For this review, take the finished solid that the model builds, in its own axes (mm). Coordinates: 2 decimals unless noted, no trailing zeros. Put each result on its own line as item: value. Start each with the question number.
Item 1: The part is to be moulded in two halves that separate along Z. For faces 1 (the flat face through (126, 4, -137)), 2 (the conical face through (49.11, 1.7, -162.32)), say which applies: +Z half, -Z half, draft (parallel to the pull), parting line (faces both ways), or undercut.
Item 2: To check wall thickness, follow L1, parallel to X at y = 0.85, z = -165; L2, parallel to X at y = 1.75, z = -135; L3, parallel to Z at x = 113, y = 0.6. State the ranges of each line that lie inside material, in increasing order.
Item 3: Insertion check: P1, Ø5, axis at x = 208, z = -165, coming from the +Y side. The pin has a flat end and moves straight along its axis. Give the tip position at first contact, or say it passes through.
```python
from build123d import *

# Parameters (mm, degrees)
SKETCH1_W                                      = 256
SKETCH1_H                                      = 270
BOSS_EXTRUDE1_DEPTH                            = 4
CSK_FOR_M5_FLAT_HEAD_MACHINE_SCREW1_AT_2_COUNT = 2
CSK_FOR_M5_FLAT_HEAD_MACHINE_SCREW1_AT_2_PITCH = 124.197423484
CSK_FOR_M5_FLAT_HEAD_MACHINE_SCREW1_AT_3_COUNT = 2
CSK_FOR_M5_FLAT_HEAD_MACHINE_SCREW1_AT_3_PITCH = 103.07764064
M6_TAPED_HOLE_THRMOCOUPLER_D                   = 5


with BuildPart() as part:
    # Sketch1 → Boss-Extrude1 (new body)
    with BuildSketch(Plane(origin=(0, 0, 0), x_dir=(1, 0, 0), z_dir=(0, 1, 0))):
        with Locations((128, 135)):
            Rectangle(SKETCH1_W, SKETCH1_H)
    extrude(amount=BOSS_EXTRUDE1_DEPTH)

    # Sketch2 → CSK for M5 Flat Head Machine Screw1 (revolve, cut)
    with BuildSketch(Plane(origin=(113, 4, -85), x_dir=(0, 0, 1), z_dir=(1, 0, 0))):
        Polygon((0, 0), (0, 4), (2.75, 4), (2.75, 2.45), (5.2, 0), align=None)
    csk_for_m5_flat_head_machine_screw1 = revolve(axis=Axis((113, 10.35, -85), (0, -1, 0)), mode=Mode.SUBTRACT)

    # CSK for M5 Flat Head Machine Screw1 at 2: CSK for M5 Flat Head Machine Screw1 ×2
    with Locations(*[Vector(0.7649111981170511, 0, -0.6441357457827795) * (i * CSK_FOR_M5_FLAT_HEAD_MACHINE_SCREW1_AT_2_PITCH) for i in range(1, CSK_FOR_M5_FLAT_HEAD_MACHINE_SCREW1_AT_2_COUNT)]):
        add(csk_for_m5_flat_head_machine_screw1, mode=Mode.SUBTRACT)

    # CSK for M5 Flat Head Machine Screw1 at 3: CSK for M5 Flat Head Machine Screw1 ×2
    with Locations(*[Vector(-0.6305926250944657, 0, -0.7761140001162656) * (i * CSK_FOR_M5_FLAT_HEAD_MACHINE_SCREW1_AT_3_PITCH) for i in range(1, CSK_FOR_M5_FLAT_HEAD_MACHINE_SCREW1_AT_3_COUNT)]):
        add(csk_for_m5_flat_head_machine_screw1, mode=Mode.SUBTRACT)

    # M6 taped hole - thrmocoupler (through all)
    with Locations(Plane(origin=(0, 4, 0), x_dir=(-1, 0, 0), z_dir=(0, 1, 0))):
        with Locations((-128, -135)):
            Hole(M6_TAPED_HOLE_THRMOCOUPLER_D / 2)


solid = part.part
```
Return value:
1. face 1: draft
1. face 2: undercut
2. L1: 0 to 45.25, 50.75 to 205.25, 210.75 to 256
2. L2: 0 to 125.5, 130.5 to 256
2. L3: -270 to -87.75, -82.25 to 0
3. P1: through
